Could you check a few things on this drawing? It's one solid part, dimensions in mm from its lowest x, y, z. Give positions to 0.01 mm unless a question says otherwise; leave off trailing zeros. Order: outer loops, then holes, each group sorted by start corner. A loop starts at its lowest first (then second) coordinate and runs counter-clockwise, first axis right, second up. Notation, with made-up numbers: (35.5, 28.5) -> (94.5, 28.5) arc R6 ccw to (94.5, 35.5) -> close; hole circle Ø1 at (57, 36.25). An arc over 180 degrees is marked (long way). Write each question's results on one line, items separated by ' | '.
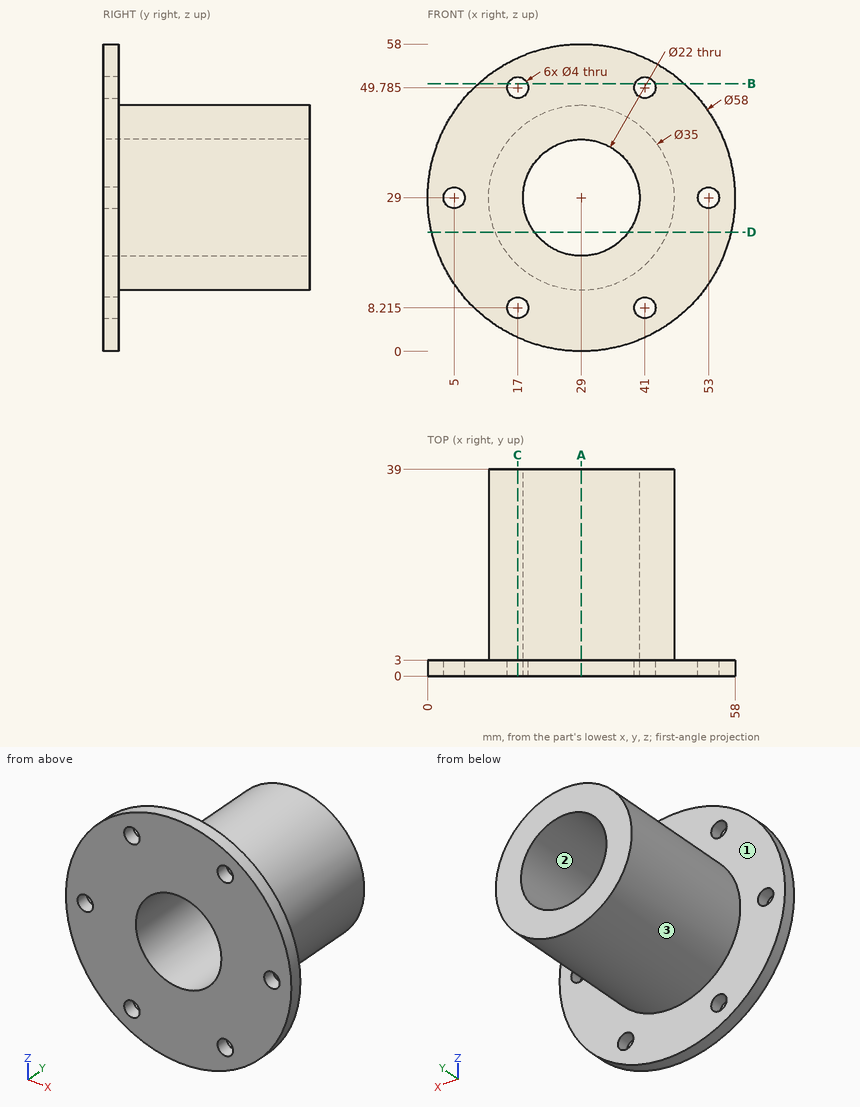
Q1. Thinking about a two-plate mould opening in Z: for the marked faces 1, 2 and 3, which applies, +Z half, -Z half, draft (parallel to the pull), parting line (faces both ways), or undercut?
Here are the results:
face 1: draft | face 2: undercut | face 3: parting line
Q2. Suppose I cut it at C-C on x = 17. Please give me the cut outline in (y, z) (1 decimal), and give its area (3 significant figures).
Here are the results:
outline: (0, 2.6) -> (3, 2.6) -> (3, 6.2) -> (0, 6.2) -> close; (0, 10.2) -> (3, 10.2) -> (3, 16.3) -> (39, 16.3) -> (39, 41.7) -> (3, 41.7) -> (3, 47.8) -> (0, 47.8) -> close; (0, 51.8) -> (3, 51.8) -> (3, 55.4) -> (0, 55.4) -> close | area: 1,050 mm²
Q3. I'm going to push flat-ended pins straight in: pin 1 Ø8 at (y, z) = (16, 17) entering from +X (1 decimal); pin 2 Ø1.5 at (x, y) = (32.5, 25) entering from -Z; pin 3 Ø10 at (x, z) = (44, 12) entering from +Y. Where does each tip first touch, or does it pass through?
Here are the results:
pin 1: stops at x = 44.6 | pin 2: stops at z = 11.72 | pin 3: stops at y = 3
Q4. Suppose I cut it at B-B on z = 50.5. Please give me the cut outline in (x, y).
Here are the results:
outline: (9.54, 0) -> (15.13, 0) -> (15.13, 3) -> (9.54, 3) -> close; (18.87, 0) -> (39.13, 0) -> (39.13, 3) -> (18.87, 3) -> close; (42.87, 0) -> (48.46, 0) -> (48.46, 3) -> (42.87, 3) -> close
Q5. I need wall thicknesses on line 1 along X through (y, z) = (2.25, 29); line 2 along Y through (x, z) = (40, 14); line 3 along Z through (x, y) = (31, 28.5) (1 decimal). Which ranges of each line are inside material? Lowest first, please.
Here are the results:
line 1: x = 0 to 3, 7 to 18, 40 to 51, 55 to 58 | line 2: y = 0 to 3 | line 3: z = 11.6 to 18.2, 39.8 to 46.4
Q6. Suppose I cut it at A-A on x = 29. Please give me the cut outline in (y, z), and give its area (3 significant figures).
Here are the results:
outline: (0, 0) -> (3, 0) -> (3, 11.5) -> (39, 11.5) -> (39, 18) -> (0, 18) -> close; (0, 40) -> (39, 40) -> (39, 46.5) -> (3, 46.5) -> (3, 58) -> (0, 58) -> close | area: 576 mm²
Q7. Suppose I cut it at D-D on z = 22.5. Please give me the cut outline in (x, y), and give its area (3 significant figures).
Here are the results:
outline: (0.74, 0) -> (20.13, 0) -> (20.13, 39) -> (12.75, 39) -> (12.75, 3) -> (0.74, 3) -> close; (37.87, 0) -> (57.26, 0) -> (57.26, 3) -> (45.25, 3) -> (45.25, 39) -> (37.87, 39) -> close | area: 647 mm²
